The listing builds one solid part. Answer for the finished solid, in the listing's coordinates (mm). Face numbers are marked on the shaded views. Round coordinates to 2 decimals unless told otherwise and drop trailing zeros. Write each loop counter-clockwise with the first axis right and the second up, starting at its lowest first coordinate (ties: lowest second). Pieces come first, ordered by that corner, then holes.
Item 1: Find the intervals of material crossed by probe 1 along X at (y, z) = (0.5, -0.85); probe 2 along Y at (x, z) = (0.5, -1.15); probe 3 along Z at (x, y) = (1.3, 1.25), in increasing order.
Item 2: Find section A-A on z = 0.95. Give the vertices of the cut face in (x, y).
Item 3: For a pull along X with two mould halves and no side action, classify the marked faces 1, 2, 3 and 4 as +X half, -X half, draft (parallel to the pull), parting line (faces both ways), or undercut.
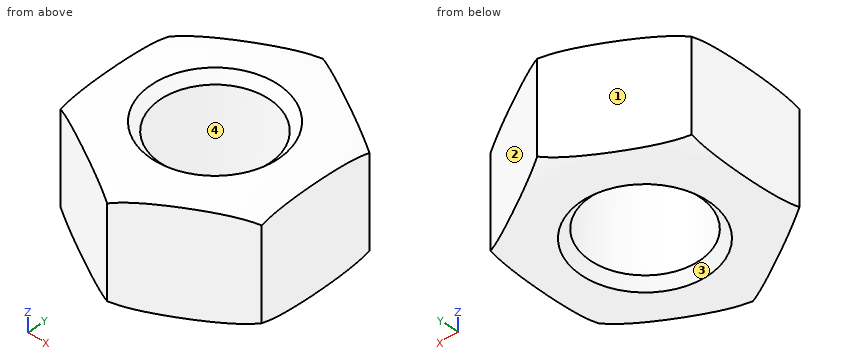
```python
from build123d import *

# Parameters (mm, degrees)
F0_R     = 1.5
F1_DEPTH = 1.5
F2_SIZE  = 0.25
F3_SIZE  = 0.25


with BuildPart() as f1:
    # F0 (on Top) → F1 (new body, symmetric)
    with BuildSketch(Plane.XY):
        Polygon((2.75, -1.5877132403), (2.75, 1.5877132403), (0, 3.1754264805), (-2.75, 1.5877132403), (-2.75, -1.5877132403), (0, -3.1754264805), align=None)
        Circle(F0_R, mode=Mode.SUBTRACT)
    extrude(amount=F1_DEPTH, both=True)

    # F2
    f2_edges = [f1.edges().sort_by_distance(p)[0] for p in [
        (-1.5, 0, 1.5),
    ]]
    chamfer(f2_edges, length=F2_SIZE)

    # F3
    f3_edges = [f1.edges().sort_by_distance(p)[0] for p in [
        (-1.5, 0, -1.5),
    ]]
    chamfer(f3_edges, length=F3_SIZE)

    # F4 (on Right) → F5 (revolve, cut)
    with BuildSketch(Plane.YZ):
        with BuildLine():
            Line((0, 1.9006831571), (0, 1.5064009931))
            add(Edge.make_bspline(
                [(0, 1.5064009931), (1.5686472961, 1.5189287501), (1.4849199585, 1.48103808), (3.2688938081, 1.4612684026), (3.4663493279, 0.9027514607)],
                knots=[0, 0, 0, 0, 0.5303558422, 1, 1, 1, 1], degree=3))
            Line((3.4663493279, 0.9027514607), (3.4663493279, -0.9027514607))
            add(Edge.make_bspline(
                [(0, -1.5064009931), (1.5686472961, -1.5189287501), (1.4849199585, -1.48103808), (3.2688938081, -1.4612684026), (3.4663493279, -0.9027514607)],
                knots=[0, 0, 0, 0, 0.5303558422, 1, 1, 1, 1], degree=3))
            Line((0, -1.5064009931), (0, -1.8480797298))
            Line((0, -1.8480797298), (4.1224174201, -1.8480797298))
            Line((4.1224174201, -1.8480797298), (4.1224174201, 1.9006831571))
            Line((4.1224174201, 1.9006831571), (0, 1.9006831571))
        make_face()
    revolve(axis=Axis((0, 0, 0), (0, 0, -1)), mode=Mode.SUBTRACT)


solid = f1.part
```
Check values:
1. probe 1: x = -2.75 to -1.41, 1.41 to 2.75
1. probe 2: y = -2.89 to -1.41, 1.41 to 2.89
1. probe 3: z = -1.49 to 1.49
2. outline: (-2.75, -1.59) - (0, -3.18) - (2.75, -1.59) - (2.75, 1.59) - (0, 3.18) - (-2.75, 1.59) - close; hole circle Ø3 at (0, 0)
3. face 1: -X half
3. face 2: +X half
3. face 3: undercut
3. face 4: undercut
